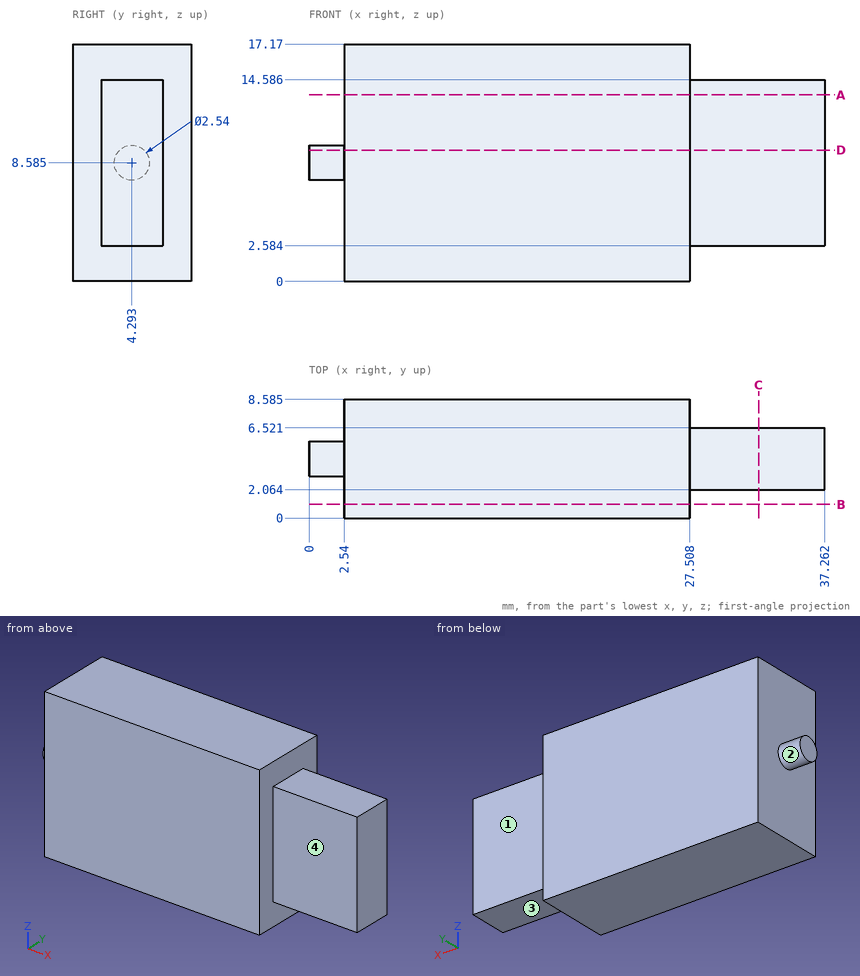
Job drawing, mm, ordinate dimensions from the low corner. One solid piece. A direction names the side the tool comes from. Give positions to 0.01 mm unless a question says otherwise; leave off trailing zeros. Loops run counter-clockwise (first coordinate to the right, second up) from the corner with the lowest first, then second, coordinate; pieces in that order, holes last. Notation, with made-up numbers: (-11.75, -25.5) -> (19.25, -25.5) arc R16 ccw to (19.25, 0.5) -> close; hole circle Ø2 at (65.25, -16). An arc over 180 degrees is marked (long way). Use a Markdown table: item, result. Add a question column.
(1) Slice it at D-D on z = 9.5. List the corners of the cut face in (x, y) (1 decimal).
(2) Slice it at B-B on y = 1. List the corners of the cut face in (x, z).
(3) Wall check: line 1 along Z through (x, y) = (28.5, 5) (1 decimal); line 2 along Y through (x, z) = (31.5, 12.25); line 3 along X through (y, z) = (4.5, 11.5). Give the ranges that are in metal, low to high.
(4) Slice it at A-A on z = 13.5. List the corners of the cut face in (x, y) (1 decimal).
(5) Slice it at C-C on x = 32.5. List the corners of the cut face in (y, z) (1 decimal), and give its area (3 significant figures).
(6) Tool access for the marked faces 1, 2, 3 and 4: list every direction of +Z, -Z, +X, -X, +Y, -Y with a clear straight run to the whole face (end or side of a thin tool).
(7) Drop flat-ended pins along their axis: pin 1 Ø5 at (x, z) = (30.5, 6.5) entering from +Y; pin 2 Ø2 at (x, y) = (35, 4.5) entering from +Z; pin 3 Ø3.5 at (x, y) = (33.5, 4) entering from -Z. Give the stop position or say it passes through.
Filled sheet:
| question | item | result |
|---|---|---|
| 1 | outline | (0, 3.4) -> (2.5, 3.4) -> (2.5, 0) -> (27.5, 0) -> (27.5, 2.1) -> (37.3, 2.1) -> (37.3, 6.5) -> (27.5, 6.5) -> (27.5, 8.6) -> (2.5, 8.6) -> (2.5, 5.2) -> (0, 5.2) -> close |
| 2 | outline | (2.54, 0) -> (27.51, 0) -> (27.51, 17.17) -> (2.54, 17.17) -> close |
| 3 | line 1 | 2.6 to 14.6 |
| 3 | line 2 | 2.06 to 6.52 |
| 3 | line 3 | 2.54 to 37.26 |
| 4 | outline | (2.5, 0) -> (27.5, 0) -> (27.5, 2.1) -> (37.3, 2.1) -> (37.3, 6.5) -> (27.5, 6.5) -> (27.5, 8.6) -> (2.5, 8.6) -> close |
| 5 | outline | (2.1, 2.6) -> (6.5, 2.6) -> (6.5, 14.6) -> (2.1, 14.6) -> close |
| 5 | area | 53.5 mm2 |
| 6 | face 1 | +Z, -Z, +X, +Y |
| 6 | face 2 | -X |
| 6 | face 3 | -Z, +X, +Y, -Y |
| 6 | face 4 | +Z, -Z, +X, -Y |
| 7 | pin 1 | y = 6.52 |
| 7 | pin 2 | z = 14.59 |
| 7 | pin 3 | z = 2.58 |
